Here's how the part is built. I have some questions about the finished solid (model axes, mm). A direction names the side the tool comes from. Round coordinates to 2 decimals unless told otherwise and drop trailing zeros. Loops run counter-clockwise (first coordinate to the right, second up) from the corner with the lowest first, then second, coordinate; pieces in that order, holes last. Notation, with made-up numbers: M -10.5,26.5 L 32.5,26.5 A20 ccw 32.5,57.5 Z; hole C 54.25,87 d10. An arc over 180 degrees is marked long. Answer as a JSON object with one key per item and string values.
Autodesk Inventor part; units mm, degrees
ref_plane "YZ Plane" through (0, 0, 0) normal (1, 0, 0) x (0, 1, 0)
ref_plane "XZ Plane" through (0, 0, 0) normal (0, 1, 0) x (-1, 0, 0)
ref_plane "XY Plane" through (0, 0, 0) normal (0, 0, 1) x (1, 0, 0)
sketch "Sketch1" plane through (0, 0, 0) normal (0, 0, 1) x (1, 0, 0)
  line L0 (-750, 39) -> (750, 39)
  line L1 (750, 39) -> (750, 0)
  line L2 (750, 0) -> (-750, 0)
  line L3 (-750, 0) -> (-750, 39)
  point P0 (0, 0)
  point P1 (0, 0)
  dimension "d0" = 1500
  dimension "d1" = 39
extrude "Plate1" add sketch "Sketch1" along normal blind 2
sketch "Sketch2" plane through (750, 2, 0) normal (0, -1, 0) x (1, 0, 0)
  line L0 (-1500, 0) -> (0, 0)
  line L1 (0, 0) -> (0, 20)
  line L2 (0, 20) -> (-1500, 20)
  line L3 (-1500, 20) -> (-1500, 0)
edge flange "Flange1" height 20 angle 90 thickness 2 bend radius 2.75 thickness toward (0, -1, 0) relief round relief width 2 relief depth 1 edges at (0, 0, 2) wall of the first edge with corners at (-750, 2, 0) (750, 2, 0) (750, 2, 20) (-750, 2, 20)
bend "Bend1"
corner "Corner1"
sketch "Sketch5" plane through (0, 0, 0) normal (0, 0, -1) x (-1, 0, 0)
  line L0 (750, 39) -> (-750, 39)
  line L1 (-1, 20) -> (-1, 39)
  line L2 (750, 0) -> (-750, 0)
  line L3 (-1, 20) -> (1, 20)
  line L4 (1, 20) -> (1, 39)
  point P0 (0, 0)
  point P1 (0, 20)
  point P2 (0, 0)
  dimension "d27" = 2
  dimension "d28" = 20
extrude "Extrusion1" cut sketch "Sketch5" against normal through all
pattern_linear "Rectangular Pattern1" count 3 spacing 500 along (1, 0, 0) of "Extrusion1" first direction both ways yes
sketch "Sketch6" plane through (0, 0, 0) normal (0, 0, -1) x (-1, 0, 0)
  line L0 (-750, 39) -> (-750, 4.75)
  circle A0 centre (-750, 39) radius 22.5
  line L1 (-750, 39) -> (750, 39)
  line L2 (-1, 39) -> (-1, 20)
  line L3 (-499, 39) -> (-499, 20)
  line L4 (-1, 20) -> (-499, 20) construction
  circle A1 centre (-250, 39) radius 22.5
  point P0 (0, 0)
  point P1 (-727.5, 39)
  point P2 (-750, 16.5)
  point P3 (-250, 20)
  dimension "d24" = 45
extrude "Extrusion2" cut sketch "Sketch6" along normal mid plane 30 contours L1 A0 L0 | A1 L1 | L1 A1 picked at (-748.3311, 24.188)
mirror "Mirror1" about plane through (0, 0, 0) normal (1, 0, 0) of "Extrusion2"
sketch "Sketch7" plane through (0, 0, 2) normal (0, 0, 1) x (1, 0, 0)
  arc A0 (-750, 16.5) -> (-727.5, 39) centre (-750, 39) ccw
  line L0 (-750, 4.75) -> (-750, 16.5)
  line L1 (-750, 4.75) -> (750, 4.75)
  line L2 (750, 16.5) -> (750, 4.75)
  arc A1 (727.5, 39) -> (750, 16.5) centre (750, 39) ccw
  line L3 (501, 39) -> (727.5, 39)
  line L4 (501, 39) -> (501, 20)
  line L5 (501, 20) -> (499, 20)
  line L6 (499, 20) -> (499, 39)
  line L7 (1, 39) -> (227.5, 39)
  line L8 (1, 39) -> (1, 20)
  line L9 (1, 20) -> (-1, 20)
  line L10 (-1, 20) -> (-1, 39)
  line L11 (-499, 39) -> (-272.5, 39)
  line L12 (-499, 39) -> (-499, 20)
  line L13 (-499, 20) -> (-501, 20)
  line L14 (-501, 20) -> (-501, 39)
  line L15 (-727.5, 39) -> (-501, 39)
  line L16 (650, 4.75) -> (650, 39) construction
  line L17 (-750, 4.75) -> (750, 4.75)
  circle A2 centre (650, 21.875) radius 5
  circle A3 centre (630, 21.875) radius 5
  line L18 (272.5, 39) -> (499, 39)
  arc A4 (227.5, 39) -> (272.5, 39) centre (250, 39) ccw
  line L19 (-227.5, 39) -> (-1, 39)
  arc A5 (-272.5, 39) -> (-227.5, 39) centre (-250, 39) ccw
  point P0 (0, 0)
  dimension "d29" = 100
  dimension "d30" = 10
  dimension "d31" = 10
  dimension "d32" = 20
extrude "Extrusion3" [suppressed]
mirror "Mirror2" [suppressed]
sketch "Sketch8" plane through (0, 0, 2) normal (0, 0, 1) x (1, 0, 0)
  line L0 (494, 34) -> (494, 22) construction
  line L1 (494, 22) -> (294, 22) construction
  line L2 (294, 22) -> (294, 34) construction
  line L3 (294, 34) -> (494, 34) construction
  line L4 (501, 39) -> (727.5, 39)
  line L5 (272.5, 39) -> (499, 39)
  point P0 (0, 0)
  dimension "d35" = 200
  dimension "d36" = 12
  dimension "d39" = 5
  dimension "d40" = 5
mark "Mark1"
equation "\"d1\" = БОРТ_стрингер_4_высота"
equation "\"d27\" = d18"
equation "\"d2\" = Thickness"
equation "\"d3\" = BendReliefWidth"
equation "\"d4\" = BendReliefDepth"
equation "\"d5\" = MinimumRemnant"
equation "\"d6\" = TransitionRadius"
equation "\"d9\" = BendRadius"
equation "\"d10\" = CornerReliefSize"
equation "\"d11\" = GapSize"
equation "\"d12\" = JacobiRadiusSize"
equation "\"BendReliefWidth\" = Thickness"
equation "\"BendReliefDepth\" = 0.5 * Thickness"
equation "\"CornerReliefSize\" = 4 * Thickness"
equation "\"MinimumRemnant\" = 2 * Thickness"
equation "\"TransitionRadius\" = BendRadius"
equation "\"JacobiRadiusSize\" = BendRadius"
equation "\"GapSize\" = Thickness"
equation "\"d18\" = Thickness"
properties part number "MSC 317 stringer board ##" material "Stainless Steel"
Item 1: For P1, Ø5, axis at x = 182.5, y = 14, coming from the -Z side; P2, Ø0.6, axis at y = 28.5, z = 1, coming from the +X side; P3, Ø1.6, axis at x = 0, z = 1.5, coming from the +Y side; P4, Ø3, axis at x = -504, y = 28, coming from the +Z side, each with a flat end and sliding along its axis, tell me the tip position at first contact or that it passes through.
Solution:
{"P1": "stops at z = 0", "P2": "stops at x = 730.26", "P3": "stops at y = 20", "P4": "stops at z = 2"}
Item 2: If I drill on L1, parallel to Z at x = 312, y = 33; L2, parallel to Y at x = 667.5, z = 1.75; L3, parallel to Z at x = 256.5, y = 4, over which ranges is the centre line in solid material (lowest first)? Write a range as from..to.
Solution:
{"L1": "z = 0..2", "L2": "y = 1.07..39", "L3": "z = 0.06..2.1"}
Item 3: I want a section at C-C on z = 12. List the corners of the cut face in (x, y) for me.
Solution:
{"outline": "M -750,0 L 750,0 L 750,2 L -750,2 Z"}
Item 4: For faces 1 (the face through (-10, 22, 0)), 2 (the face through (-10, 22, 2)), which set-ups out of +Z, -Z, +X, -X, +Y, -Y let a thin tool reach every point of the face, with its end or its side?
Solution:
{"face 1": "-Z, +X, -X, +Y, -Y", "face 2": "+Z, +X, -X, +Y"}
Item 5: I want a section at B-B on x = -643.5. List the corners of the cut face in (y, z) for me, plus the area to 3 significant figures.
Solution:
{"outline": "M 0,4.75 A4.75 ccw 4.75,0 L 39,0 L 39,2 L 4.75,2 A2.75 cw 2,4.75 L 2,20 L 0,20 Z", "area": "111 mm2"}
Item 6: I want a section at A-A on x = -250. List the corners of the cut face in (y, z) for me, plus the area to 3 significant figures.
Solution:
{"outline": "M 0,4.75 A4.75 ccw 4.75,0 L 16.5,0 L 16.5,2 L 4.75,2 A2.75 cw 2,4.75 L 2,20 L 0,20 Z", "area": "65.8 mm2"}
